Input: part model. Units: mm. Frame: model coordinates. A direction names the side the tool comes from. Coordinates: 2 decimals unless noted, no trailing zeros. Order: outer loops, then holes, each group sorted by start corner. A loop starts at its lowest first (then second) coordinate and runs counter-clockwise, first axis right, second up. Notation, with made-up numbers: M 63,2.25 L 78,2.25 A17 cw 78,9.25 Z; hole C 26.25,10 d6. An arc over 180 degrees is marked long. One line per item, written item: value.
```python
from build123d import *

# Parameters (mm, degrees)
SKETCH_1_W           = 166
SKETCH_1_H           = 138
EXTRUDE_1_DEPTH      = 2
EXTRUDE_2_DEPTH      = 6
EXTRUDE_2_DEPTH_BACK = 8
SKETCH_2_W           = 158
SKETCH_2_H           = 130
SKETCH_2_W_2         = 154
SKETCH_2_H_2         = 126
SKETCH_3_R           = 1.5
EXTRUDE_2_2_DEPTH    = 5
SKETCH_5_R           = 1.5
EXTRUDE_3_DEPTH      = 5
SKETCH_4_R           = 1.5
EXTRUDE_4_DEPTH      = 5
SKETCH_6_W           = 75
SKETCH_6_H           = 2
SKETCH_6_W_2         = 2
SKETCH_6_H_2         = 75
EXTRUDE_5_DEPTH      = 8
SKETCH_9_W           = 90
SKETCH_9_H           = 2
EXTRUDE_6_DEPTH      = 1
FILLET_1_R           = 1
SKETCH_11_W          = 90
SKETCH_11_H          = 2
EXTRUDE_7_DEPTH      = 1
FILLET_2_R           = 1


with BuildPart() as part:
    # 스케치1 → 보스-돌출1 (new body)
    with BuildSketch(Plane.XY):
        Rectangle(SKETCH_1_W, SKETCH_1_H)
    extrude(amount=EXTRUDE_1_DEPTH)

    # 스케치2 → Extrude 2 (add, two sides: drawn at the far end of the back side and taken through both)
    with BuildSketch(Plane.XY.offset(2).offset(-EXTRUDE_2_DEPTH_BACK)):
        Rectangle(SKETCH_2_W, SKETCH_2_H)
        Rectangle(SKETCH_2_W_2, SKETCH_2_H_2, mode=Mode.SUBTRACT)
    extrude(amount=EXTRUDE_2_DEPTH + EXTRUDE_2_DEPTH_BACK)

    # 스케치3 → Extrude 2 2 (add)
    with BuildSketch(Plane.XY.offset(2)):
        with Locations(Location((-65, -42, 0), (0, 0, 180))):
            Circle(SKETCH_3_R)
        with Locations(Location((-50, -42, 0), (0, 0, 180))):
            Circle(SKETCH_3_R)
        with Locations(Location((-65, 42, 0), (0, 0, 180))):
            Circle(SKETCH_3_R)
        with Locations(Location((-50, 42, 0), (0, 0, 180))):
            Circle(SKETCH_3_R)
    extrude(amount=EXTRUDE_2_2_DEPTH)

    # 스케치5 → 보스-돌출3 (add)
    with BuildSketch(Plane.XY.offset(2)):
        with Locations(Location((42, 56, 0), (0, 0, 180))):
            Circle(SKETCH_5_R)
        with Locations(Location((42, 41, 0), (0, 0, 180))):
            Circle(SKETCH_5_R)
    extrude(amount=EXTRUDE_3_DEPTH)

    # 스케치4 → 보스-돌출4 (add)
    with BuildSketch(Plane.XY.offset(2)):
        with Locations(Location((-42, 56, 0), (0, 0, 180))):
            Circle(SKETCH_4_R)
        with Locations(Location((-42, 41, 0), (0, 0, 180))):
            Circle(SKETCH_4_R)
    extrude(amount=EXTRUDE_4_DEPTH)

    # 스케치6 → 보스-돌출5 (add)
    with BuildSketch(Plane.XY.offset(2)):
        with Locations((0, -54)):
            Rectangle(SKETCH_6_W, SKETCH_6_H)
        with Locations((0, -44)):
            Rectangle(SKETCH_6_W, SKETCH_6_H)
        with Locations((46, 0)):
            Rectangle(SKETCH_6_W_2, SKETCH_6_H_2)
        with Locations((56, 0)):
            Rectangle(SKETCH_6_W_2, SKETCH_6_H_2)
    extrude(amount=EXTRUDE_5_DEPTH)

    # 스케치9 → 보스-돌출6 (add)
    with BuildSketch(Plane.XZ.offset(65)):
        with Locations((0, 5)):
            Rectangle(SKETCH_9_W, SKETCH_9_H)
    extrude(amount=EXTRUDE_6_DEPTH)

    # 필렛1
    fillet_1_edges = [part.edges().sort_by_distance(p)[0] for p in [
        (0, -66, 4),
        (0, -66, 6),
    ]]
    fillet(fillet_1_edges, radius=FILLET_1_R - 0.0001)  # a hair under: the kernel refuses the full size

    # 스케치11 → 보스-돌출7 (add)
    with BuildSketch(Plane(origin=(0, 65, 0), x_dir=(1, 0, 0), z_dir=(0, 1, 0))):
        with Locations((0, -5)):
            Rectangle(SKETCH_11_W, SKETCH_11_H)
    extrude(amount=EXTRUDE_7_DEPTH)

    # 필렛2
    fillet_2_edges = [part.edges().sort_by_distance(p)[0] for p in [
        (0, 66, 4),
        (0, 66, 6),
    ]]
    fillet(fillet_2_edges, radius=FILLET_2_R - 0.0001)  # a hair under: the kernel refuses the full size


solid = part.part
```
(1) Draft query along Y for faces 4 (the flat face through (-7, -66, 0)), 5 (the flat face through (47, -1, 6)), 6 (the flat face through (-77, -1, -3)), 7 (the flat face through (-1, -65, -3)). Return one class per face: released by +Y, released by -Y, zero draft, split by the parting line, or undercut.
Data:
face 4: zero draft
face 5: undercut
face 6: undercut
face 7: released by -Y
(2) Ray query, line 1 (Y direction, x = 36, z = 7); line 2 (X direction, y = -22, z = -5); line 3 (Y direction, x = 54, z = 7.5). Return the intervals inside material, ascending. Write a range as from..to.
Data:
line 1: y = -65..-63, -55..-53, -45..-43, 63..65
line 2: x = -79..-77, 77..79
line 3: y = -65..-63, 63..65
(3) Cut plane C-C on y = -58. Output: boundary loops of the cut face in (x, z).
Data:
outline: M -83,0 L -79,0 L -79,-6 L -77,-6 L -77,0 L 77,0 L 77,-6 L 79,-6 L 79,0 L 83,0 L 83,2 L 79,2 L 79,8 L 77,8 L 77,2 L -77,2 L -77,8 L -79,8 L -79,2 L -83,2 Z
(4) Access query for faces 1 (the flat face through (-79, -1, -3)), 2 (the flat face through (-1, 63, 5)), 3 (the flat face through (-1, 1, 0)). Directions: +Z, -Z, +X, -X, +Y, -Y. A direction counts if a zero-diameter tool reaches every point of the face in a straight line with its end or side. Return the directions, or none.
Data:
face 1: -Z, -X, +Y, -Y
face 2: +Z
face 3: -Z
(5) Cut plane B-B on x = 53. Output: boundary loops of the cut face in (y, z), plus the area to 3 significant figures.
Data:
outline: M -69,0 L -65,0 L -65,-6 L -63,-6 L -63,0 L 63,0 L 63,-6 L 65,-6 L 65,0 L 69,0 L 69,2 L 65,2 L 65,8 L 63,8 L 63,2 L -63,2 L -63,8 L -65,8 L -65,2 L -69,2 Z
area: 324 mm2
(6) First-contact query: pin 1 (3 mm diameter, centred on x = 33, z = 5.5, fed in from -Y); pin 2 (4 mm diameter, centred on y = -8.5, z = 6.5, fed in from -X); pin 3 (3 mm diameter, centred on x = -8, z = 5, fed in from +Y); pin 4 (8 mm diameter, centred on y = -18, z = 3, fed in from +X). Flat tips, straight axial feed; report the tip coordinate or a pass-through.
Data:
pin 1: stops at y = -66
pin 2: stops at x = -79
pin 3: stops at y = 66
pin 4: stops at x = 83
(7) Cut plane A-A on y = 20. Output: boundary loops of the cut face in (x, z), plus the area to 3 significant figures.
Data:
outline: M -83,0 L -79,0 L -79,-6 L -77,-6 L -77,0 L 77,0 L 77,-6 L 79,-6 L 79,0 L 83,0 L 83,2 L 79,2 L 79,8 L 77,8 L 77,2 L 57,2 L 57,10 L 55,10 L 55,2 L 47,2 L 47,10 L 45,10 L 45,2 L -77,2 L -77,8 L -79,8 L -79,2 L -83,2 Z
area: 412 mm2
